The listing builds one solid part. Answer for the finished solid, in the listing's coordinates (mm). A direction names the side the tool comes from. Give positions to 0.01 mm unless a question says otherwise; leave off trailing zeros. Order: outer loops, then holes, each group sorted by start corner. A loop starts at its lowest first (then second) coordinate and runs counter-clockwise, first axis right, second up. Notation, with made-up numbers: (-6, 32.5) - (42, 32.5) arc R33 ccw to (42, 71.5) - close; hole circle Ø5 at (-21, 29). An arc over 180 degrees is marked (long way). Answer as a JSON object with one key per item and string values. Group by question number.
Q1. The mould has two halves that part along Y. Classify faces 1 (the face through (58, 24, -13)), 2 (the face through (56, 0, -55)), 3 (the face through (60, 0, -3)): released by +Y, released by -Y, zero draft, split by the parting line, or undercut.
Q2. A cutting plane is placed at B-B, the plane x = 50. Give the vertices of the cut face in (y, z), and give its area (3 significant figures).
Q3. A cutting plane is placed at D-D, the plane x = 27.5. Give the vertices of the cut face in (y, z), and give its area (3 significant figures).
Q4. Given pin 1 (5 mm diameter, centred on x = 10, y = 22.5, fed in from +Z); pin 2 (3 mm diameter, centred on x = 39.5, y = 6.5, fed in from +Z); pin 3 (1 mm diameter, centred on x = 31.5, y = 16.5, fed in from +Z), each flat-ended and moving along its own axis, determine where each tip first touches the part or whether it passes through.
Q5. For faces 4 (the face through (58, 0, -50)), 5 (the face through (58, -24, -12)), determine the directions among +Z, -Z, +X, -X, +Y, -Y from which every point of the face is accessible in a straight line to the end or side of a thin tool.
Q6. A cutting plane is placed at A-A, the plane y = 0. Give the vertices of the cut face in (x, z), and give its area (3 significant figures).
Q7. A cutting plane is placed at C-C, the plane z = -11. Give the vertices of the cut face in (x, y).
Q8. Consider line 1 (Y direction, x = 50, z = -55.5); line 2 (Y direction, x = 44, z = -48); line 3 (X direction, y = 10, z = 0). Determine where each line is inside the solid, lowest interval first.
from build123d import *

# Parameters (mm, degrees)
BOSS_EXTRUDE1_DEPTH = 60
CUT_EXTRUDE1_REACH  = 90.459
SKETCH2_R           = 7.5
SKETCH3_W           = 50
SKETCH3_H           = 40
CUT_EXTRUDE2_DEPTH  = 70
SKETCH4_R           = 1.5
CUT_EXTRUDE3_DEPTH  = 10
FILLET2_R           = 5


with BuildPart() as part:
    # Sketch1 → Boss-Extrude1 (new body)
    with BuildSketch(Plane(origin=(0, 0, 0), x_dir=(0, 0, -1), z_dir=(1, 0, 0))):
        with BuildLine():
            Line((-35, 25), (60, 25))
            Line((60, 25), (60, -25))
            Line((60, -25), (-35, -25))
            ThreePointArc((-35, -25), (-60, 0), (-35, 25))
        make_face()
    extrude(amount=BOSS_EXTRUDE1_DEPTH)

    # Sketch2 → Cut-Extrude1 (cut, up to next)
    with BuildSketch(Plane(origin=(60, 0, 0), x_dir=(0, 0, -1), z_dir=(1, 0, 0)), mode=Mode.PRIVATE) as cut_extrude1_sk1:
        with Locations((-35, 0)):
            Circle(SKETCH2_R)
    cut_extrude1_tool1 = extrude(cut_extrude1_sk1.sketch, amount=-CUT_EXTRUDE1_REACH, mode=Mode.PRIVATE) & part.part
    add(cut_extrude1_tool1.solids().sort_by_distance((60, 0, 35))[0], mode=Mode.SUBTRACT)

    # Sketch3 → Cut-Extrude2 (cut)
    with BuildSketch(Plane(origin=(0, 0, -60), x_dir=(-1, 0, 0), z_dir=(0, 0, -1))):
        with Locations((-30, 0)):
            Rectangle(SKETCH3_W, SKETCH3_H)
    extrude(amount=-CUT_EXTRUDE2_DEPTH, mode=Mode.SUBTRACT)

    # Sketch4 → Cut-Extrude3 (cut)
    with BuildSketch(Plane(origin=(0, 0, -60), x_dir=(-1, 0, 0), z_dir=(0, 0, -1))):
        with Locations((-50, 22.5)):
            Circle(SKETCH4_R)
        with Locations((-50, -22.5)):
            Circle(SKETCH4_R)
        with Locations((-10, -22.5)):
            Circle(SKETCH4_R)
        with Locations((-10, 22.5)):
            Circle(SKETCH4_R)
        with Locations((-57.5, 0)):
            Circle(SKETCH4_R)
        with Locations((-2.5, 0)):
            Circle(SKETCH4_R)
    extrude(amount=-CUT_EXTRUDE3_DEPTH, mode=Mode.SUBTRACT)

    # Fillet2
    fillet2_edges = [part.edges().sort_by_distance(p)[0] for p in [
        (60, 25, -12.5),
        (60, 0, 60),
        (0, 25, -12.5),
        (0, -25, -12.5),
        (0, 0, 60),
        (60, -25, -12.5),
    ]]
    fillet(fillet2_edges, radius=FILLET2_R)


solid = part.part
Reply:
{
 "1": {"face 1": "released by +Y", "face 2": "undercut", "face 3": "zero draft"},
 "2": {"outline": "(-25, -60) - (-24, -60) - (-24, -50) - (-21, -50) - (-21, -60) - (-20, -60) - (-20, 10) - (20, 10) - (20, -60) - (21, -60) - (21, -50) - (24, -50) - (24, -60) - (25, -60) - (25, 35) arc R25 ccw to (-25, 35) - close; hole circle Ø15 at (0, 35)", "area": "2,700 mm^2"},
 "3": {"outline": "(-25, -60) - (-20, -60) - (-20, 10) - (20, 10) - (20, -60) - (25, -60) - (25, 35) arc R25 ccw to (-25, 35) - close; hole circle Ø15 at (0, 35)", "area": "2,760 mm^2"},
 "4": {"pin 1": "stops at z = 50", "pin 2": "stops at z = 59.49", "pin 3": "stops at z = 54.21"},
 "5": {"face 4": "-Z", "face 5": "+Z, -Z, +X, -Y"},
 "6": {"outline": "(0, -60) - (1, -60) - (1, -50) - (4, -50) - (4, -60) - (5, -60) - (5, 10) - (55, 10) - (55, -60) - (56, -60) - (56, -50) - (59, -50) - (59, -60) - (60, -60) - (60, 27.5) - (0, 27.5) - close; (0, 42.5) - (60, 42.5) - (60, 55) arc R5 ccw to (55, 60) - (5, 60) arc R5 ccw to (0, 55) - close", "area": "2,730 mm^2"},
 "7": {"outline": "(0, -20) arc R5 ccw to (5, -25) - (55, -25) arc R5 ccw to (60, -20) - (60, 20) arc R5 ccw to (55, 25) - (5, 25) arc R5 ccw to (0, 20) - close; hole (5, -20) - (55, -20) - (55, 20) - (5, 20) - close"},
 "8": {"line 1": "y = -25 to -24, -21 to -20, 20 to 21, 24 to 25", "line 2": "y = -25 to -20, 20 to 25", "line 3": "x = 0 to 5, 55 to 60"}
}
